Geometry check sheet. Reference: the model listing, model coordinates, mm. Face numbers are marked on the shaded views. A direction names the side the tool comes from. Coordinates: 2 decimals unless noted, no trailing zeros. Order: outer loops, then holes, each group sorted by start corner. A loop starts at its lowest first (then second) coordinate and runs counter-clockwise, first axis right, second up. Notation, with made-up numbers: (4, 88.5) - (44, 88.5) arc R15 ccw to (44, 112.5) - close; hole circle Ø11 at (10.5, 71). An arc over 180 degrees is marked (long way). Use CSV: the item, a comma, the result in double quotes. Start each with the question number.
1) Thickness scan on probe 1 along Z at (x, y) = (7.5, -10.25); probe 2 along X at (y, z) = (-9, 17); probe 3 along Y at (x, z) = (8.5, 0). Record the ranges inside material, lowest first. Write a range as [from, to].
2) Tool access check on the marked faces 5, 6 and 7. Record the directions out of +Z, -Z, +X, -X, +Y, -Y that give a thin tool (end or side, any length) a straight path to the whole face; none if there is none.
3) Sectioned sample at B-B, the plane z = 0. Record the cut outline in (x, y).
4) Sectioned sample at C-C, the plane y = 6.5. Record the cut outline in (x, z), and give its area (3 significant figures).
5) Sectioned sample at A-A, the plane x = 8.25. Record the cut outline in (y, z), and give its area (3 significant figures).
6) Sectioned sample at D-D, the plane x = 10.5. Record the cut outline in (y, z), and give its area (3 significant figures).
7) Draft check along Z on the marked faces 1, 2, 3 and 4. Enter one of: released by +Z, released by -Z, zero draft, split by the parting line, or undercut.
8) Depth check by flat-ended pin: P1, Ø5, axis at x = 10.5, z = -18.5, coming from the +Y side; P2, Ø4.5, axis at x = 6.5, y = 3, coming from the -Z side; P3, Ø7.5, axis at x = 9, z = 16, coming from the +Y side; P4, Ø1.5, axis at y = 16.5, z = -5, coming from the +X side. Enter the tip coordinate at first touch or a pass-through.
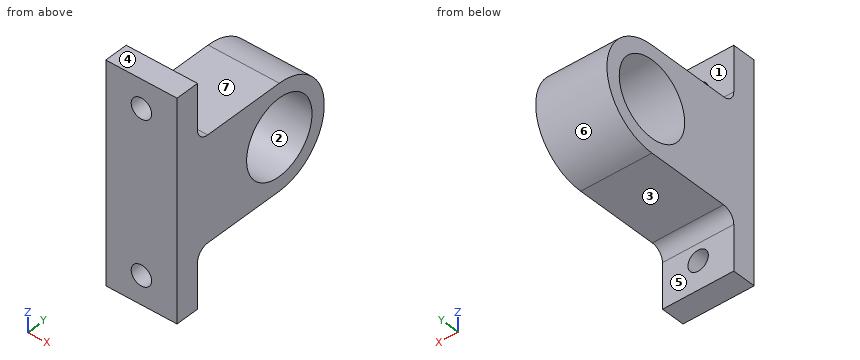
from build123d import *

# Parameters (mm, degrees)
SKETCH1_R                = 8
BOSS_EXTRUDE1_DEPTH      = 15
SKETCH2_W                = 15
SKETCH2_H                = 5
BOSS_EXTRUDE2_DEPTH      = 12
BOSS_EXTRUDE2_DEPTH_BACK = 34
SKETCH3_R                = 2.15
CUT_EXTRUDE1_DEPTH       = 5
FILLET1_R                = 2.5


with BuildPart() as part:
    # Sketch1 → Boss-Extrude1 (new body)
    with BuildSketch(Plane(origin=(0, 0, 0), x_dir=(0, 0, -1), z_dir=(1, 0, 0))):
        with BuildLine():
            Line((-11, 12.5), (-11, -12.5))
            Line((-11, -12.5), (11, -12.5))
            Line((11, -12.5), (11, 12.5))
            ThreePointArc((11, 12.5), (0, 23.5), (-11, 12.5))
        make_face()
        with Locations((0, 12.5)):
            Circle(SKETCH1_R, mode=Mode.SUBTRACT)
    extrude(amount=BOSS_EXTRUDE1_DEPTH)

    # Sketch2 → Boss-Extrude2 (add, two sides)
    with BuildSketch(Plane.XY.offset(11)) as boss_extrude2_sk:
        with Locations((7.5, -10)):
            Rectangle(SKETCH2_W, SKETCH2_H)
    extrude(amount=BOSS_EXTRUDE2_DEPTH)
    extrude(boss_extrude2_sk.sketch, amount=-BOSS_EXTRUDE2_DEPTH_BACK)

    # Sketch3 → Cut-Extrude1 (cut)
    with BuildSketch(Plane(origin=(0, -7.5, 0), x_dir=(1, 0, 0), z_dir=(0, 1, 0))):
        with Locations((7.5, -17)):
            Circle(SKETCH3_R)
        with Locations((7.5, 17)):
            Circle(SKETCH3_R)
    extrude(amount=-CUT_EXTRUDE1_DEPTH, mode=Mode.SUBTRACT)

    # Fillet1
    fillet1_edges = [part.edges().sort_by_distance(p)[0] for p in [
        (7.5, -7.5, 11),
        (7.5, -7.5, -11),
    ]]
    fillet(fillet1_edges, radius=FILLET1_R)


solid = part.part
Evaluation:
1,probe 1,"[-23, -19.15], [-14.85, 14.85], [19.15, 23]"
1,probe 2,"[0, 5.35], [9.65, 15]"
1,probe 3,"[-12.5, 4.5], [20.5, 23.5]"
2,face 5,"-Z, +X, -X, +Y"
2,face 6,"+X, -X, +Y"
2,face 7,"+Z, +X, -X, +Y"
3,outline,"(0, -12.5) - (15, -12.5) - (15, 4.5) - (0, 4.5) - close; (0, 20.5) - (15, 20.5) - (15, 23.5) - (0, 23.5) - close"
4,outline,"(0, -11) - (15, -11) - (15, -5.29) - (0, -5.29) - close; (0, 5.29) - (15, 5.29) - (15, 11) - (0, 11) - close"
4,area,"171 mm²"
5,outline,"(-12.5, -23) - (-7.5, -23) - (-7.5, -19.01) - (-12.5, -19.01) - close; (-12.5, -14.99) - (-7.5, -14.99) - (-7.5, -13.5) arc R2.5 cw to (-5, -11) - (12.5, -11) arc R11 ccw to (12.5, 11) - (-5, 11) arc R2.5 cw to (-7.5, 13.5) - (-7.5, 14.99) - (-12.5, 14.99) - close; (-12.5, 19.01) - (-7.5, 19.01) - (-7.5, 23) - (-12.5, 23) - close; hole circle Ø16 at (12.5, 0)"
5,area,"621 mm²"
6,outline,"(-12.5, -23) - (-7.5, -23) - (-7.5, -13.5) arc R2.5 cw to (-5, -11) - (12.5, -11) arc R11 ccw to (12.5, 11) - (-5, 11) arc R2.5 cw to (-7.5, 13.5) - (-7.5, 23) - (-12.5, 23) - close; hole circle Ø16 at (12.5, 0)"
6,area,"662 mm²"
7,face 1,"zero draft"
7,face 2,"undercut"
7,face 3,"released by -Z"
7,face 4,"released by +Z"
8,P1,"y = -7.5"
8,P2,"z = -11"
8,P3,"y = -7.17"
8,P4,"through"
